Work out the finished part from the listing and answer in its coordinate system (mm). A direction names the side the tool comes from. Give positions to 0.01 mm unless a question says otherwise; leave off trailing zeros. Loops run counter-clockwise (first coordinate to the right, second up) from the corner with the lowest first, then second, coordinate; pieces in that order, holes last. Notation, with made-up numbers: M 33,-36.5 L 46,-36.5 A15 ccw 46,-18.5 Z; hole C 52.5,66.25 d6. An arc over 180 degrees is marked long. Answer as a JSON object with one key per item and string values. Group by question number.
```python
from build123d import *

# Parameters (mm, degrees)
SKETCH1_W               = 16
SKETCH1_H               = 16
BOSS_EXTRUDE1_DEPTH     = 24
SKETCH12_W              = 12.4
SKETCH12_H              = 12.4
CUT_EXTRUDE6_DEPTH      = 22
SKETCH13_R              = 20
BOSS_EXTRUDE2_DEPTH     = 3
CHAMFER1_SIZE           = 2.5
SKETCH14_W              = 16
SKETCH14_H              = 16
BOSS_EXTRUDE3_DEPTH     = 12
CUT_EXTRUDE1_DEPTH      = 7.5
SKETCH11_W              = 4.2
SKETCH11_H              = 5.5
CUT_EXTRUDE5_DEPTH      = 6.3
CUT_EXTRUDE5_DEPTH_BACK = 0.1
CHAMFER2_SIZE           = 2
CHAMFER4_SIZE           = 2
SKETCH15_R              = 1.3
CUT_EXTRUDE7_DEPTH      = 28.5
CHAMFER5_SIZE           = 1


with BuildPart() as part:
    # Sketch1 → Boss-Extrude1 (new body)
    with BuildSketch(Plane(origin=(0, 0, 0), x_dir=(1, 0, 0), z_dir=(0, 1, 0))):
        with Locations((0, 8)):
            Rectangle(SKETCH1_W, SKETCH1_H)
    extrude(amount=BOSS_EXTRUDE1_DEPTH)

    # Sketch12 → Cut-Extrude6 (cut)
    with BuildSketch(Plane(origin=(0, 24, 0), x_dir=(1, 0, 0), z_dir=(0, 1, 0))):
        with Locations((0, 8)):
            Rectangle(SKETCH12_W, SKETCH12_H)
    extrude(amount=-CUT_EXTRUDE6_DEPTH, mode=Mode.SUBTRACT)

    # Sketch13 → Boss-Extrude2 (add)
    with BuildSketch(Plane(origin=(0, 0, 0), x_dir=(1, 0, 0), z_dir=(0, 1, 0))):
        with Locations((0, 8)):
            Circle(SKETCH13_R)
    extrude(amount=BOSS_EXTRUDE2_DEPTH)

    # Chamfer1
    chamfer1_edges = [part.edges().sort_by_distance(p)[0] for p in [
        (-20, 3, -8),
    ]]
    chamfer(chamfer1_edges, length=CHAMFER1_SIZE)

    # Sketch14 → Boss-Extrude3 (add)
    with BuildSketch(Plane(origin=(0, 3, 0), x_dir=(1, 0, 0), z_dir=(0, 1, 0))):
        Polygon((-8, 23), (8, 23), (9, 23), (9, -4), (8, -4), (-8, -4), (-9, -4), (-9, 23), align=None)
        with Locations((0, 8)):
            Rectangle(SKETCH14_W, SKETCH14_H, mode=Mode.SUBTRACT)
    extrude(amount=BOSS_EXTRUDE3_DEPTH)

    # Sketch5 → Cut-Extrude1 (cut)
    with BuildSketch(Plane(origin=(0, 0, -23), x_dir=(-1, 0, 0), z_dir=(0, 0, -1))):
        with BuildLine():
            Line((-2.1, 11.1), (2.1, 11.1))
            Line((2.1, 11.1), (3.1, 10.1))
            Line((3.1, 10.1), (3.1, 8.8))
            ThreePointArc((3.1, 8.8), (3.9, 8), (3.1, 7.2))
            Line((3.1, 7.2), (3.1, 4.9))
            Line((3.1, 4.9), (-3.1, 4.9))
            Line((-3.1, 4.9), (-3.1, 7.2))
            ThreePointArc((-3.1, 7.2), (-3.9, 8), (-3.1, 8.8))
            Line((-3.1, 8.8), (-3.1, 10.1))
            Line((-3.1, 10.1), (-2.1, 11.1))
        make_face()
    extrude(amount=-CUT_EXTRUDE1_DEPTH, mode=Mode.SUBTRACT)

    # Sketch11 → Cut-Extrude5 (cut, two sides)
    with BuildSketch(Plane.XZ.offset(-11.1)) as cut_extrude5_sk:
        with Locations((0, -18.25)):
            Rectangle(SKETCH11_W, SKETCH11_H)
    extrude(amount=CUT_EXTRUDE5_DEPTH, mode=Mode.SUBTRACT)
    extrude(cut_extrude5_sk.sketch, amount=-CUT_EXTRUDE5_DEPTH_BACK, mode=Mode.SUBTRACT)

    # Chamfer2
    chamfer2_edges = [part.edges().sort_by_distance(p)[0] for p in [
        (0, 15, -23),
        (9, 9, -23),
        (-9, 9, -23),
    ]]
    chamfer(chamfer2_edges, length=CHAMFER2_SIZE)

    # Chamfer4
    chamfer4_edges = [part.edges().sort_by_distance(p)[0] for p in [
        (0, 15, 4),
        (-9, 9, 4),
        (9, 9, 4),
    ]]
    chamfer(chamfer4_edges, length=CHAMFER4_SIZE)

    # Sketch15 → Cut-Extrude7 (cut, through all)
    with BuildSketch(Plane(origin=(0, 0, -15.5), x_dir=(-1, 0, 0), z_dir=(0, 0, -1))):
        with Locations((0, 8)):
            Circle(SKETCH15_R)
    extrude(amount=-CUT_EXTRUDE7_DEPTH, mode=Mode.SUBTRACT)

    # Chamfer5
    chamfer5_edges = [part.edges().sort_by_distance(p)[0] for p in [
        (0, 24, -16),
        (-8, 24, -8),
        (0, 24, 0),
        (8, 24, -8),
    ]]
    chamfer(chamfer5_edges, length=CHAMFER5_SIZE)


solid = part.part
```
Item 1: For a pull along Z with two mould halves and no side action, classify faces 1 (the flat face through (6.2, 14, -8)), 2 (the conical face through (-13.984, 2.879, 2.722)), 3 (the flat face through (0, 19, 0)) as pulls with the +Z half, pulls with the -Z half, needs draft (parallel to the pull), parting line crosses it, or undercut.
Item 2: A cutting plane is placed at B-B (z = -8). Determine the outline of the cut face in (x, y).
Item 3: A cutting plane is placed at C-C (y = 3.75). Determine the outline of the cut face in (x, z), and give its area (3 significant figures).
Item 4: A tool of negligible diameter and unlimited length cuts with its end or side. For faces 4 (the flat face through (0, 19, -16)), 5 (the flat face through (8, 9, -22)), 6 (the flat face through (-6.2, 14, -8)), from which of +Z, -Z, +X, -X, +Y, -Y can it reach the whole face along a straight path? Write none if from no direction.
Item 5: Given pin 1 Ø9 at (x, y) = (0, 18) entering from -Z; pin 2 Ø3.5 at (x, y) = (2.5, 12.5) entering from -Z; pin 3 Ø0.6 at (y, z) = (9.5, -17.5) entering from -X, each flat-ended and moving along its own axis, determine where each tip first touches the part or whether it passes through.
Item 6: A cutting plane is placed at D-D (x = 0). Give the number of separate pieces and of enclosed holes in the cut face, and give its area (3 significant figures).
Item 7: A cutting plane is placed at A-A (y = 8). Determine the outline of the cut face in (x, z), and give its area (3 significant figures).
Item 8: Find the intervals of material crossed by probe 1 along Y at (x, z) = (0, 1); probe 2 along Y at (x, z) = (1.5, -18.5); probe 3 along Z at (x, y) = (4, 8.5), in increasing order. Write a range as [from, to].
The answers:
{
 "1": {"face 1": "undercut", "face 2": "parting line crosses it", "face 3": "pulls with the +Z half"},
 "2": {"outline": "M -20,0 L 20,0 L 20,0.5 L 17.5,3 L 9,3 L 9,15 L 8,15 L 8,23 L 7,24 L 6.2,24 L 6.2,3 L -6.2,3 L -6.2,24 L -7,24 L -8,23 L -8,15 L -9,15 L -9,3 L -17.5,3 L -20,0.5 Z"},
 "3": {"outline": "M -9,-21 L -7,-23 L 7,-23 L 9,-21 L 9,2 L 7,4 L -7,4 L -9,2 Z; hole M -6.2,-14.2 L 6.2,-14.2 L 6.2,-1.8 L -6.2,-1.8 Z", "area": "324 mm^2"},
 "4": {"face 4": "-Z, +X, -X, +Y", "face 5": "-Z, +X, +Y", "face 6": "+Y"},
 "5": {"pin 1": "stops at z = -22.5", "pin 2": "stops at z = -23", "pin 3": "stops at x = -9"},
 "6": {"separate pieces": "3", "enclosed holes": "0", "area": "250 mm^2"},
 "7": {"outline": "M -9,-21 L -7,-23 L -3.9,-23 L -3.9,-15.5 L -1.3,-15.5 L -1.3,-14.2 L -6.2,-14.2 L -6.2,-1.8 L -1.3,-1.8 L -1.3,4 L -7,4 L -9,2 Z; M 1.3,-15.5 L 3.9,-15.5 L 3.9,-23 L 7,-23 L 9,-21 L 9,2 L 7,4 L 1.3,4 L 1.3,-1.8 L 6.2,-1.8 L 6.2,-14.2 L 1.3,-14.2 Z", "area": "247 mm^2"},
 "8": {"probe 1": "y = [0, 6.7], [9.3, 15]", "probe 2": "y = [0, 4.8], [11.2, 15]", "probe 3": "z = [-23, -14.2], [-1.8, 4]"}
}
